Work out the finished part from the listing and answer in its coordinate system (mm). A direction names the side the tool comes from. Round coordinates to 2 decimals unless told otherwise and drop trailing zeros. Write each loop counter-clockwise with the first axis right and the second up, starting at its lowest first coordinate (ties: lowest second). Pieces come first, ordered by that corner, then holes. Notation, with made-up numbers: (8, 21) -> (34, 21) arc R17 cw to (34, 43) -> close; hole circle Ø6 at (17.25, -31). An arc over 180 degrees is marked (long way). One line per question, with ' | ' between items. Start each with the question number.
```python
from build123d import *

# Parameters (mm, degrees)
SKETCH1_R               = 13.75
BOSS_EXTRUDE1_DEPTH     = 4
BOSS_EXTRUDE2_START     = 4
SKETCH5_R               = 8.5
BOSS_EXTRUDE2_DEPTH     = 4
CUT_EXTRUDE1_DEPTH      = 22.026768653
CUT_EXTRUDE1_DEPTH_BACK = 22.026768653
SKETCH6_W               = 2.888681075
SKETCH6_H               = 2.039823556
SKETCH6_W_2             = 2.682346713
SKETCH8_R               = 7
CUT_EXTRUDE3_DEPTH      = 12


with BuildPart() as part:
    # Sketch1 → Boss-Extrude1 (new body)
    with BuildSketch(Plane(origin=(0, 0, 0), x_dir=(1, 0, 0), z_dir=(0, 1, 0))):
        with Locations(Location((0, 0, 0), (0, 0, 270))):
            Circle(SKETCH1_R)
    extrude(amount=BOSS_EXTRUDE1_DEPTH)

    # Sketch5 → Boss-Extrude2 (add)
    with BuildSketch(Plane(origin=(0, 0, 0), x_dir=(1, 0, 0), z_dir=(0, 1, 0)).offset(BOSS_EXTRUDE2_START)):
        with Locations(Location((0, 0, 0), (0, 0, 270))):
            Circle(SKETCH5_R)
    extrude(amount=BOSS_EXTRUDE2_DEPTH)

    # Sketch6 → Cut-Extrude1 (cut, two sides: drawn at the far end of the back side and taken through both)
    with BuildSketch(Plane.XY.offset(-CUT_EXTRUDE1_DEPTH_BACK)):
        with Locations((-9.95563299, 2)):
            Rectangle(SKETCH6_W, SKETCH6_H)
        with Locations((10.007216581, 2)):
            Rectangle(SKETCH6_W_2, SKETCH6_H)
    extrude(amount=CUT_EXTRUDE1_DEPTH + CUT_EXTRUDE1_DEPTH_BACK, mode=Mode.SUBTRACT)

    # Sketch8 → Cut-Extrude3 (cut)
    with BuildSketch(Plane(origin=(0, 0, 0), x_dir=(1, 0, 0), z_dir=(0, 1, 0))):
        with Locations(Location((0, 0, 0), (0, 0, 270))):
            Circle(SKETCH8_R)
    extrude(amount=CUT_EXTRUDE3_DEPTH, mode=Mode.SUBTRACT)


solid = part.part
```
(1) The mould has two halves that part along Z. Classify faces 4 (the flat face through (7, 8, 2)), 5 (the cylindrical face through (-12.2, 1.97, 6.34)), 6 (the cylindrical face through (-6.834, 3.944, -1.517)): +Z half, -Z half, draft (parallel to the pull), parting line (faces both ways), or undercut.
(2) A cutting plane is placed at C-C, the plane y = 1.5. Determine the outline of the cut face in (x, z), then the cut area to 3 significant figures.
(3) A cutting plane is placed at A-A, the plane z = 0. Determine the outline of the cut face in (x, y).
(4) A cutting plane is placed at B-B, the plane x = 0. Determine the outline of the cut face in (y, z).
(5) Consider L1, parallel to X at y = 1.75, z = 0; L2, parallel to Y at x = 11, z = -0.25; L3, parallel to X at y = 5.75, z = 0. Determine where each line is inside the solid, lowest interval first.
(6) Given pin 1 Ø3 at (x, y) = (9, 2) entering from -Z; pin 2 Ø0.6 at (y, z) = (1.5, -2) entering from -X; pin 3 Ø1.4 at (x, z) = (-10.5, 0) entering from +Y, each flat-ended and moving along its own axis, determine where each tip first touches the part or whether it passes through.
(7) A cutting plane is placed at D-D, the plane z = -6.5. Determine the outline of the cut face in (x, y).
(8) For faces 1 (the cylindrical face through (8.428, 5.972, -1.107)), 2 (the flat face through (10, 0.98, 0)), 3 (the flat face through (-6, 0, 6)), determine the directions among +Z, -Z, +X, -X, +Y, -Y from which every point of the face is accessible in a straight line to the end or side of a thin tool.
Returned:
1) face 4: draft | face 5: parting line | face 6: undercut
2) outline: (-11.4, -7.69) -> (-11.4, 7.69) arc R13.75 ccw to start; (-8.51, -10.8) arc R13.75 ccw to (8.67, -10.68) -> (8.67, 10.68) arc R13.75 ccw to (-8.51, 10.8) -> close; (11.35, -7.76) arc R13.75 ccw to (11.35, 7.76) -> close; hole circle Ø14 at (0, 0) | area: 335 mm2
3) outline: (-13.75, 0) -> (-7, 0) -> (-7, 8) -> (-8.5, 8) -> (-8.5, 4) -> (-13.75, 4) -> close; (7, 0) -> (13.75, 0) -> (13.75, 4) -> (8.5, 4) -> (8.5, 8) -> (7, 8) -> close; hole (-11.4, 0.98) -> (-8.51, 0.98) -> (-8.51, 3.02) -> (-11.4, 3.02) -> close; hole (8.67, 0.98) -> (11.35, 0.98) -> (11.35, 3.02) -> (8.67, 3.02) -> close
4) outline: (0, -13.75) -> (4, -13.75) -> (4, -8.5) -> (8, -8.5) -> (8, -7) -> (0, -7) -> close; (0, 7) -> (8, 7) -> (8, 8.5) -> (4, 8.5) -> (4, 13.75) -> (0, 13.75) -> close
5) L1: -13.75 to -11.4, -8.51 to -7, 7 to 8.67, 11.35 to 13.75 | L2: 0 to 0.98, 3.02 to 4 | L3: -8.5 to -7, 7 to 8.5
6) pin 1: z = -11.52 | pin 2: x = -13.64 | pin 3: y = 4
7) outline: (-12.12, 0) -> (-2.6, 0) -> (-2.6, 8) -> (-5.48, 8) -> (-5.48, 4) -> (-12.12, 4) -> close; (2.6, 0) -> (12.12, 0) -> (12.12, 4) -> (5.48, 4) -> (5.48, 8) -> (2.6, 8) -> close; hole (-11.4, 0.98) -> (-8.51, 0.98) -> (-8.51, 3.02) -> (-11.4, 3.02) -> close; hole (8.67, 0.98) -> (11.35, 0.98) -> (11.35, 3.02) -> (8.67, 3.02) -> close
8) face 1: +Y | face 2: +Z, -Z | face 3: +Z, -Z, +X, -X, -Y
